Answer from the drawing. Dimensions are ordinates in mm from the lowest x, y and z of the part. Give positions to 0.01 mm unless a question says otherwise; leave off trailing zeros. Write each loop counter-clockwise with the first axis right and the second up, starting at its lowest first coordinate (ties: lowest second). Pieces come first, ordered by that corner, then holes.
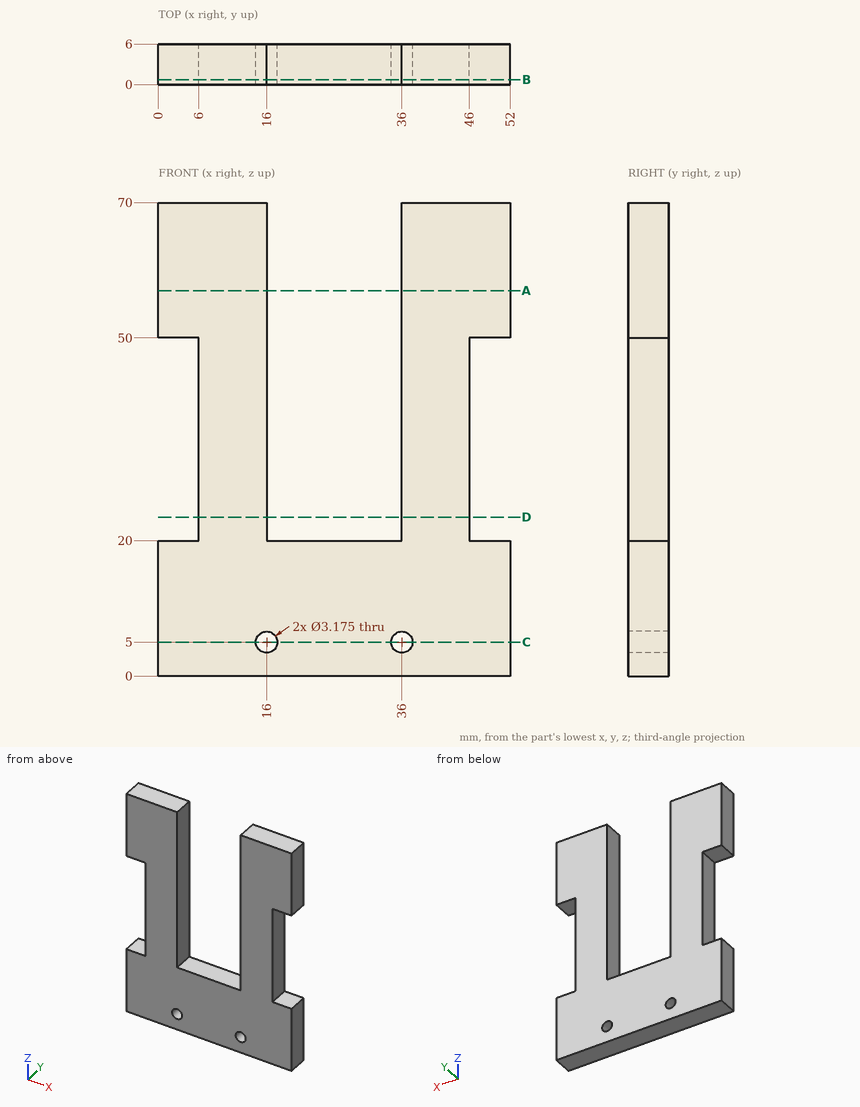
Item 1: Consider probe 1 along X at (y, z) = (3.5, 5); probe 2 along X at (y, z) = (3.1, 29); probe 3 along X at (y, z) = (0.65, 61). Determine where each line is inside the solid, lowest interval first.
Conclusion:
probe 1: x = 0 to 14.41, 17.59 to 34.41, 37.59 to 52
probe 2: x = 6 to 16, 36 to 46
probe 3: x = 0 to 16, 36 to 52
Item 2: Each of these flat-tipped pins is pushed along its axis until it touches: P1, Ø1.8, axis at y = 4, z = 36, coming from the +X side; P2, Ø1.8, axis at y = 3, z = 35, coming from the -X side. Where does it stop, or does it pass through?
Conclusion:
P1: stops at x = 46
P2: stops at x = 6
Item 3: A cutting plane is placed at B-B, the plane y = 0.75. Give the vertices of the cut face in (x, z) (1 decimal), plus the area to 3 significant figures.
Conclusion:
outline: (0, 0) - (52, 0) - (52, 20) - (46, 20) - (46, 50) - (52, 50) - (52, 70) - (36, 70) - (36, 20) - (16, 20) - (16, 70) - (0, 70) - (0, 50) - (6, 50) - (6, 20) - (0, 20) - close; hole circle Ø3.2 at (16, 5); hole circle Ø3.2 at (36, 5)
area: 2,260 mm2
Item 4: A cutting plane is placed at A-A, the plane z = 57. Give the vertices of the cut face in (x, y), plus the area to 3 significant figures.
Conclusion:
outline: (0, 0) - (16, 0) - (16, 6) - (0, 6) - close; (36, 0) - (52, 0) - (52, 6) - (36, 6) - close
area: 192 mm2
Item 5: A cutting plane is placed at D-D, the plane z = 23.5. Give the vertices of the cut face in (x, y), plus the area to 3 significant figures.
Conclusion:
outline: (6, 0) - (16, 0) - (16, 6) - (6, 6) - close; (36, 0) - (46, 0) - (46, 6) - (36, 6) - close
area: 120 mm2
Item 6: A cutting plane is placed at C-C, the plane z = 5. Give the vertices of the cut face in (x, y), plus the area to 3 significant figures.
Conclusion:
outline: (0, 0) - (14.41, 0) - (14.41, 6) - (0, 6) - close; (17.59, 0) - (34.41, 0) - (34.41, 6) - (17.59, 6) - close; (37.59, 0) - (52, 0) - (52, 6) - (37.59, 6) - close
area: 274 mm2
